Can you work these out from the drawing? Everything is in mm from the part's minimum corner. Coordinates: 2 decimals unless noted, no trailing zeros. Loops run counter-clockwise (first coordinate to the right, second up) from the corner with the lowest first, then second, coordinate; pieces in that order, holes last. Notation, with made-up numbers: (50.25, 53.5) - (78.25, 53.5) arc R25 ccw to (78.25, 81.5) - close; hole circle Ø9 at (-25, 57). An arc over 180 degrees is marked (long way). One line per question, with ' | ' between items. Start each with the question number.
1. I want a section at B-B, the plane y = 2.25. Write out the boundary of the cut face in (x, z).
2. I'm going to push flat-ended pins straight in: P1, Ø0.5, axis at x = 37.5, z = 21.5, coming from the -Y side; P2, Ø3, axis at y = 14, z = 10, coming from the -X side; P3, Ø2, axis at y = 16.5, z = 34.5, coming from the +X side; P4, Ø10, axis at x = 49, y = 12, coming from the -Z side. Where does each tip first touch, or does it pass through?
3. I want a section at D-D, the plane x = 12. Write out the boundary of the cut face in (y, z).
4. I want a section at A-A, the plane z = 21. Write out the boundary of the cut face in (x, y), then the cut area to 3 significant figures.
5. Please list where these lines run through material, in increasing order: L1, parallel to X at y = 1.25, z = 15; L2, parallel to X at y = 14.5, z = 21; L3, parallel to X at y = 9, z = 6. Write a range as [from, to].
6. I want a section at C-C, the plane x = 63. Write out the boundary of the cut face in (y, z), then the cut area to 3 significant figures.
7. We'd pull the mould along X, two halves only. Please class the marked faces 1 and 2: pulls with the +X half, pulls with the -X half, needs draft (parallel to the pull), parting line crosses it, or undercut.
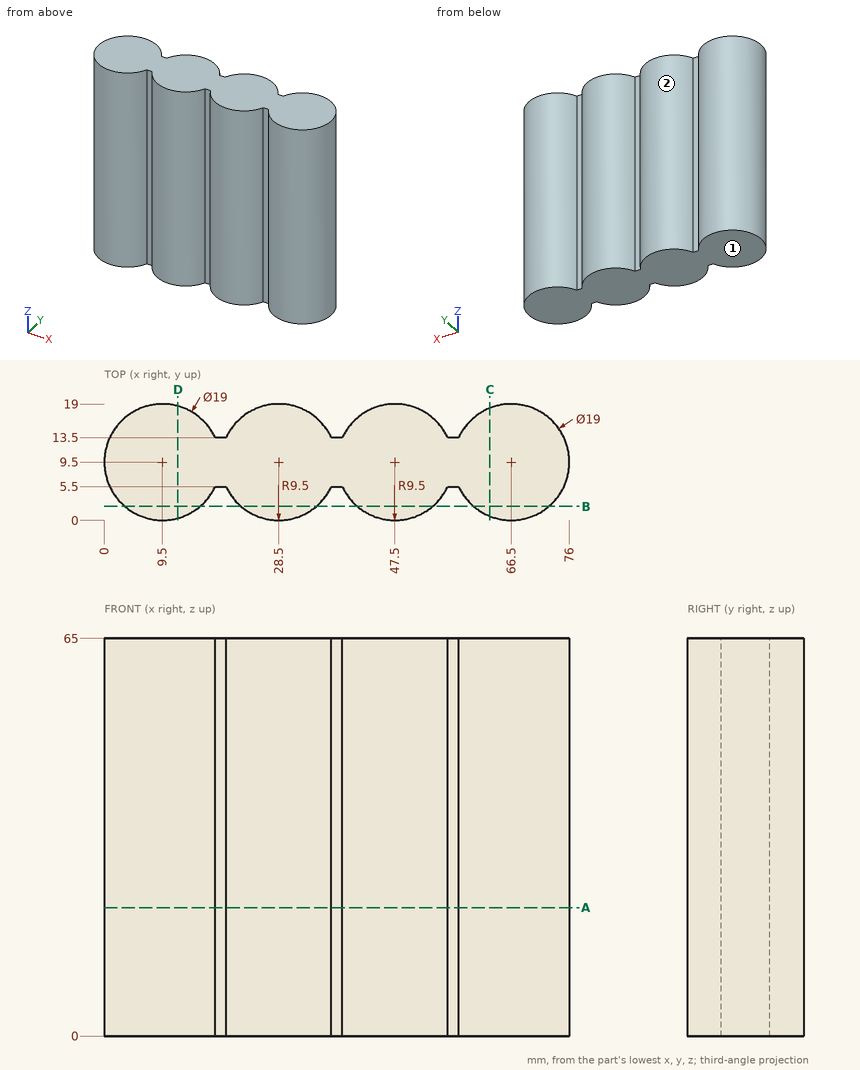
Results are:
1) outline: (3.36, 0) - (15.64, 0) - (15.64, 65) - (3.36, 65) - close; (22.36, 0) - (34.64, 0) - (34.64, 65) - (22.36, 65) - close; (41.36, 0) - (53.64, 0) - (53.64, 65) - (41.36, 65) - close; (60.36, 0) - (72.64, 0) - (72.64, 65) - (60.36, 65) - close
2) P1: stops at y = 5.5 | P2: stops at x = 0.49 | P3: stops at x = 73.87 | P4: stops at z = 0
3) outline: (0.33, 0) - (18.67, 0) - (18.67, 65) - (0.33, 65) - close
4) outline: (18.12, 5.5) - (19.88, 5.5) arc R9.5 ccw to (37.12, 5.5) - (38.88, 5.5) arc R9.5 ccw to (56.12, 5.5) - (57.88, 5.5) arc R9.5 ccw (long way) to (57.88, 13.5) - (56.12, 13.5) arc R9.5 ccw to (38.88, 13.5) - (37.12, 13.5) arc R9.5 ccw to (19.88, 13.5) - (18.12, 13.5) arc R9.5 ccw (long way) to start | area: 1,150 mm2
5) L1: x = [4.79, 14.21], [23.79, 33.21], [42.79, 52.21], [61.79, 71.21] | L2: x = [1.42, 17.58], [20.42, 36.58], [39.42, 55.58], [58.42, 74.58] | L3: x = [0.01, 75.99]
6) outline: (0.67, 0) - (18.33, 0) - (18.33, 65) - (0.67, 65) - close | area: 1,150 mm2
7) face 1: needs draft | face 2: undercut
